Part print with two shaded views. Sizes in mm from the minimum x, y, z corner. A direction names the side the tool comes from. Coordinates: 2 decimals unless noted, no trailing zeros. Write each loop counter-clockwise with the first axis right and the second up, starting at its lowest first coordinate (ties: lowest second). Pieces come first, ordered by that corner, then holes. Notation, with made-up numbers: (89.5, -23) - (128.5, -23) arc R11 cw to (128.5, -19) - close; hole circle Ø11 at (22, 58). An arc over 180 degrees is marked (long way). Answer in a Markdown table with one row per item. Add a question column.
Q1. Drill centre lines: line 1 along Y through (x, z) = (6, 0.85); line 2 along Y through (x, z) = (37, 0.9); line 3 along Y through (x, z) = (18, 8.5). Where is each one in solid material? Low to high. Write a range as from..to.
Q2. Pin check, flat tips, straight feed: pin 1 (3 mm diameter, centred on x = 6, y = 18.5, fed in from -Z); pin 2 (1.5 mm diameter, centred on x = 28.5, y = 3, fed in from +Z); pin 3 (6 mm diameter, centred on x = 26, z = 9.5, fed in from +Y); pin 4 (5 mm diameter, centred on x = 13.5, z = 8.5, fed in from -Y). Stop position of each tip, or through.
Q3. Band-saw the part on A-A (y = 18.5). List the corners of the cut face in (x, z).
Q4. 3-axis set-ups, long thin cutter, end or side, ignore diameter. For the marked faces 1, 2 and 3: which of +Z, -Z, +X, -X, +Y, -Y reach the whole face in a straight line?
Q5. Band-saw the part on C-C (x = 23). List the corners of the cut face in (y, z).
Q6. Band-saw the part on B-B (x = 6). List the corners of the cut face in (y, z), and give its area (3 significant figures).
Q7. Band-saw the part on D-D (z = 10.25). List the corners of the cut face in (x, y).
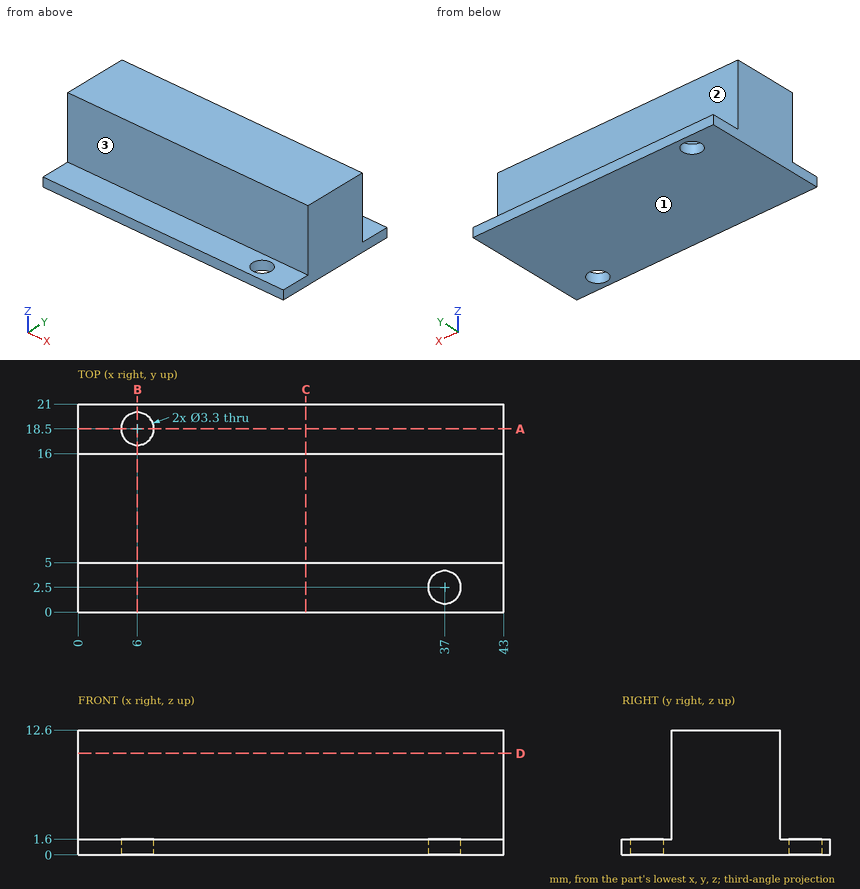
Checked values:
| question | item | result |
|---|---|---|
| 1 | line 1 | y = 0..16.85, 20.15..21 |
| 1 | line 2 | y = 0..0.85, 4.15..21 |
| 1 | line 3 | y = 5..16 |
| 2 | pin 1 | passes through |
| 2 | pin 2 | stops at z = 1.6 |
| 2 | pin 3 | stops at y = 16 |
| 2 | pin 4 | stops at y = 5 |
| 3 | outline | (0, 0) - (4.35, 0) - (4.35, 1.6) - (0, 1.6) - close; (7.65, 0) - (43, 0) - (43, 1.6) - (7.65, 1.6) - close |
| 4 | face 1 | -Z, +X, -X, +Y, -Y |
| 4 | face 2 | +Z, +X, -X, +Y |
| 4 | face 3 | +Z, +X, -X, -Y |
| 5 | outline | (0, 0) - (21, 0) - (21, 1.6) - (16, 1.6) - (16, 12.6) - (5, 12.6) - (5, 1.6) - (0, 1.6) - close |
| 6 | outline | (0, 0) - (16.85, 0) - (16.85, 1.6) - (16, 1.6) - (16, 12.6) - (5, 12.6) - (5, 1.6) - (0, 1.6) - close; (20.15, 0) - (21, 0) - (21, 1.6) - (20.15, 1.6) - close |
| 6 | area | 149 mm² |
| 7 | outline | (0, 5) - (43, 5) - (43, 16) - (0, 16) - close |
